Read the model definition and answer for the solid it produces. Units are mm, in the model's axes. A direction names the side the tool comes from. Coordinates: 2 decimals unless noted, no trailing zeros. Write each loop counter-clockwise with the first axis right and the second up, starting at its lowest first coordinate (ties: lowest second). Pieces come first, ordered by that corner, then holes. Notation, with made-up numbers: (35, 77.5) -> (78, 77.5) arc R21 cw to (78, 100.5) -> close; hole circle Ø3 at (88, -26.5). An arc over 180 degrees is marked (long way). Answer as a JSON object with one key per item and string values. Group by question number.
(1) Straight lines are drawn through the part: L1, parallel to X at y = 5.5, z = 0; L2, parallel to X at y = 3, z = 0. For each, find the intervals that lie inside material, in ascending order.
(2) Find section C-C (y = 1.4). Give the vertices of the cut face in (x, z).
(3) Flat-ended cylindrical pins translate along their axes: P1, Ø1.8, axis at x = -7.25, z = 0, coming from the +Y side; P2, Ø4, axis at x = 0, z = 0, coming from the +Y side; P3, Ø3, axis at y = 4, z = 6.5, coming from the -X side. Find the tip coordinate at first contact, or state that the pin passes through.
(4) For a pull along Z with two mould halves and no side action, classify faces 4 (the face through (3, 6, 3)), 5 (the face through (14.78, 0.49, 6.13)), 6 (the face through (-0.867, 5.014, 3.905)) as +Z half, -Z half, draft (parallel to the pull), parting line (faces both ways), or undercut.
(5) Find section A-A (z = 0). Give the vertices of the cut face in (x, y).
(6) Which of the six approach directions +Z, -Z, +X, -X, +Y, -Y give full straight-line access (tool end or side, diameter ignored) to faces 1 (the face through (2, 4, 0)), 2 (the face through (10.818, 3.573, 5.627)), 3 (the face through (-0.13, 2.96, 6.26))?
(7) Find section B-B (y = 3). Give the vertices of the cut face in (x, z).
from build123d import *

# Parameters (mm, degrees)
SKETCH1_R           = 16
SKETCH1_R_2         = 1
SKETCH1_R_3         = 1.5
BOSS_EXTRUDE1_DEPTH = 6
SKETCH2_R           = 4
CUT_EXTRUDE1_DEPTH  = 2


with BuildPart() as part:
    # Sketch1 → Boss-Extrude1 (new body)
    with BuildSketch(Plane(origin=(0, 0, 0), x_dir=(1, 0, 0), z_dir=(0, 1, 0))):
        Circle(SKETCH1_R)
        with Locations((0, 7.25)):
            Circle(SKETCH1_R_2, mode=Mode.SUBTRACT)
        with Locations((7.25, 0)):
            Circle(SKETCH1_R_2, mode=Mode.SUBTRACT)
        with Locations((0, -7.25)):
            Circle(SKETCH1_R_2, mode=Mode.SUBTRACT)
        with Locations((-7.25, 0)):
            Circle(SKETCH1_R_2, mode=Mode.SUBTRACT)
        Circle(SKETCH1_R_3, mode=Mode.SUBTRACT)
    extrude(amount=BOSS_EXTRUDE1_DEPTH)

    # Sketch2 → Cut-Extrude1 (cut)
    with BuildSketch(Plane(origin=(0, 6, 0), x_dir=(1, 0, 0), z_dir=(0, 1, 0))):
        Circle(SKETCH2_R)
    extrude(amount=-CUT_EXTRUDE1_DEPTH, mode=Mode.SUBTRACT)

    # Sketch3 → Cut-Revolve1 (revolve, cut)
    with BuildSketch(Plane(origin=(0, 0, 0), x_dir=(0, 0, -1), z_dir=(1, 0, 0))):
        Polygon((-16, 5), (-12, 3.5), (-12, 2.5), (-16, 1), align=None)
    revolve(axis=Axis((0, 6, 0), (0, -1, 0)), mode=Mode.SUBTRACT)


solid = part.part
Results below:
{
 "1": {"L1": "x = -16 to -8.25, -6.25 to -4, 4 to 6.25, 8.25 to 16", "L2": "x = -12 to -8.25, -6.25 to -1.5, 1.5 to 6.25, 8.25 to 12"},
 "2": {"outline": "circle Ø29.87 at (0, 0); hole circle Ø2 at (-7.25, 0); hole circle Ø3 at (0, 0); hole circle Ø2 at (0, -7.25); hole circle Ø2 at (0, 7.25); hole circle Ø2 at (7.25, 0)"},
 "3": {"P1": "passes through", "P2": "stops at y = 4", "P3": "stops at x = -15.07"},
 "4": {"face 4": "draft", "face 5": "parting line", "face 6": "undercut"},
 "5": {"outline": "(-16, 0) -> (-8.25, 0) -> (-8.25, 6) -> (-16, 6) -> (-16, 5) -> (-12, 3.5) -> (-12, 2.5) -> (-16, 1) -> close; (-6.25, 0) -> (-1.5, 0) -> (-1.5, 4) -> (-4, 4) -> (-4, 6) -> (-6.25, 6) -> close; (1.5, 0) -> (6.25, 0) -> (6.25, 6) -> (4, 6) -> (4, 4) -> (1.5, 4) -> close; (8.25, 0) -> (16, 0) -> (16, 1) -> (12, 2.5) -> (12, 3.5) -> (16, 5) -> (16, 6) -> (8.25, 6) -> close"},
 "6": {"face 1": "+Y", "face 2": "none", "face 3": "+Y, -Y"},
 "7": {"outline": "circle Ø24 at (0, 0); hole circle Ø2 at (-7.25, 0); hole circle Ø3 at (0, 0); hole circle Ø2 at (0, -7.25); hole circle Ø2 at (0, 7.25); hole circle Ø2 at (7.25, 0)"}
}
